Can you work these out from the model? Positions are in its coordinate system, mm. Face numbers are marked on the shaded views. Give positions to 0.01 mm unless a question says otherwise; leave off trailing zeros. Write each loop counter-clockwise with the first axis right and the second up, starting at its lowest first coordinate (ties: lowest second). Pieces come first, ordered by that corner, then holes.
1. Suppose I cut it at D-D (y = 2.5). Please give me the cut outline in (x, z), and give its area (3 significant figures).
2. If I drill on probe 1 along Z at (x, y) = (25, 4.25); probe 2 along X at (y, z) = (5.5, 2.5); probe 3 along Y at (x, z) = (29.5, 2.75), over which ranges is the centre line in solid material (lowest first)?
3. Thinking about a two-plate mould opening in Z: for the marked faces 1, 2 and 3, which applies, pulls with the +Z half, pulls with the -Z half, needs draft (parallel to the pull), parting line crosses it, or undercut?
4. Suppose I cut it at B-B (x = 25). Please give me the cut outline in (y, z), and give its area (3 significant figures).
5. Suppose I cut it at C-C (y = 9.5). Please give me the cut outline in (x, z).
6. Suppose I cut it at A-A (z = 0). Please give me the cut outline in (x, y).
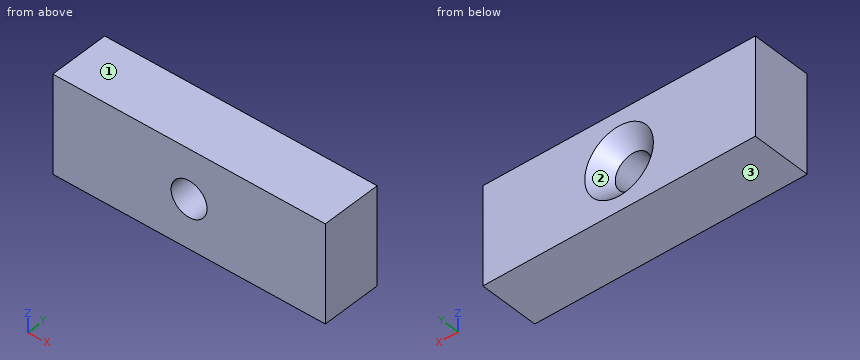
```python
from build123d import *

# Parameters (mm, degrees)
BOSS_EXTRUDE1_DEPTH                                 = 11
SKETCH2_W                                           = 10.92366107
SKETCH2_H                                           = 18
SKETCH2_W_2                                         = 14.331152634
CUT_EXTRUDE1_DEPTH                                  = 12
CSK_FOR_M6_COUNTERSUNK_FLAT_HEAD_SCREW1_D           = 6.6
CSK_FOR_M6_COUNTERSUNK_FLAT_HEAD_SCREW1_CSINK_D     = 12.6
CSK_FOR_M6_COUNTERSUNK_FLAT_HEAD_SCREW1_CSINK_ANGLE = 90


with BuildPart() as part:
    # Sketch1 → Boss-Extrude1 (new body)
    with BuildSketch(Plane(origin=(0, 0, 0), x_dir=(1, 0, 0), z_dir=(0, 1, 0))):
        with BuildLine():
            Line((0, 9), (50, 9))
            ThreePointArc((50, 9), (59, 0), (50, -9))
            Line((50, -9), (0, -9))
            ThreePointArc((0, -9), (-9, 0), (0, 9))
        make_face()
    extrude(amount=BOSS_EXTRUDE1_DEPTH)

    # Sketch2 → Cut-Extrude1 (cut, through all)
    with BuildSketch(Plane(origin=(0, 11, 0), x_dir=(1, 0, 0), z_dir=(0, 1, 0))):
        with Locations((-5.461830535, 0)):
            Rectangle(SKETCH2_W, SKETCH2_H)
        with Locations((57.165576317, 0)):
            Rectangle(SKETCH2_W_2, SKETCH2_H)
    extrude(amount=-CUT_EXTRUDE1_DEPTH, mode=Mode.SUBTRACT)

    # CSK for M6 Countersunk Flat Head Screw1 (through all)
    with Locations(Plane(origin=(0, 11, 0), x_dir=(1, 0, 0), z_dir=(0, 1, 0))):
        with Locations((25, 0)):
            CounterSinkHole(CSK_FOR_M6_COUNTERSUNK_FLAT_HEAD_SCREW1_D / 2, CSK_FOR_M6_COUNTERSUNK_FLAT_HEAD_SCREW1_CSINK_D / 2, counter_sink_angle=CSK_FOR_M6_COUNTERSUNK_FLAT_HEAD_SCREW1_CSINK_ANGLE)


solid = part.part
```
Checks:
1. outline: (0, -9) - (50, -9) - (50, 9) - (0, 9) - close; hole circle Ø6.6 at (25, 0)
1. area: 866 mm2
2. probe 1: z = -9 to -3.3, 3.3 to 9
2. probe 2: x = 0 to 22.85, 27.15 to 50
2. probe 3: y = 0 to 9.97
3. face 1: pulls with the +Z half
3. face 2: undercut
3. face 3: pulls with the -Z half
4. outline: (0, -9) - (11, -9) - (11, -6.3) - (8, -3.3) - (0, -3.3) - close; (0, 3.3) - (8, 3.3) - (11, 6.3) - (11, 9) - (0, 9) - close
4. area: 116 mm2
5. outline: (0, -9) - (50, -9) - (50, 9) - (0, 9) - close; hole circle Ø9.6 at (25, 0)
6. outline: (0, 0) - (21.7, 0) - (21.7, 8) - (18.7, 11) - (0, 11) - close; (28.3, 0) - (50, 0) - (50, 11) - (31.3, 11) - (28.3, 8) - close
